The model under review builds one solid part; all positions refer to its coordinate system, in mm. Face numbers are marked on the shaded views. Coordinates: 2 decimals unless noted, no trailing zeros. Order: outer loops, then holes, each group sorted by start corner. A loop starts at its lowest first (then second) coordinate and runs counter-clockwise, first axis right, second up. Notation, with made-up numbers: M 80.25,65 L 126.25,65 A25 ccw 126.25,94 Z; hole C 52,82.25 d10. An arc over 180 degrees is marked long. Answer as CSV lines item,"result". Start each with the question number.
Q1. The part is to be moulded in two halves that separate along X. For the marked faces 1, 2 and 3, say which applies: +X half, -X half, draft (parallel to the pull), parting line (faces both ways), or undercut.
Q2. Wall thickness on L1, parallel to Y at x = -6.75, z = 19.5; L2, parallel to Y at x = 5.5, z = 7.25; L3, parallel to Y at x = -7.75, z = 26.25: over which ranges is each line inside the solid? List them lowest first. Write a range as [from, to].
Q3. Consider section C-C on z = 8.75. Write out the cut boundary in (x, y), and give its area (3 significant figures).
Q4. Consider section A-A on y = 0. Write out the cut boundary in (x, z), and give its area (3 significant figures).
Q5. For P1, Ø1.8, axis at x = 6.72, y = -6.72, coming from the -Z side, flat-tipped, find the tip position at first contact; note if it passes through.
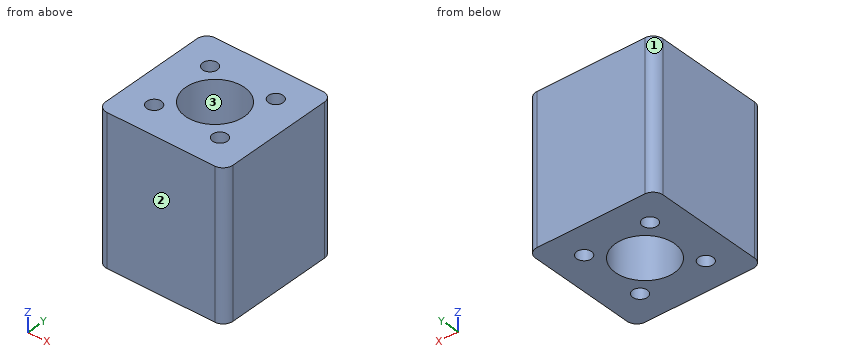
from build123d import *

# Parameters (mm, degrees)
SKETCH_1_R      = 1.5
SKETCH_1_R_2    = 6
EXTRUDE_1_DEPTH = 30


with BuildPart() as part:
    # 草图1 → 凸台-拉伸1 (new body)
    with BuildSketch(Plane.XY):
        with BuildLine():
            Line((0, 13), (11, 13))
            ThreePointArc((11, 13), (12.414213562, 12.414213562), (13, 11))
            Line((13, 11), (13, -11))
            ThreePointArc((13, -11), (12.414213562, -12.414213562), (11, -13))
            Line((11, -13), (-11, -13))
            ThreePointArc((-11, -13), (-12.414213562, -12.414213562), (-13, -11))
            Line((-13, -11), (-13, 11))
            ThreePointArc((-13, 11), (-12.414213562, 12.414213562), (-11, 13))
            Line((-11, 13), (0, 13))
        make_face()
        with Locations((-6.717514421, 6.717514421)):
            Circle(SKETCH_1_R, mode=Mode.SUBTRACT)
        with Locations((6.717514421, 6.717514421)):
            Circle(SKETCH_1_R, mode=Mode.SUBTRACT)
        with Locations((-6.717514421, -6.717514421)):
            Circle(SKETCH_1_R, mode=Mode.SUBTRACT)
        with Locations((6.717514421, -6.717514421)):
            Circle(SKETCH_1_R, mode=Mode.SUBTRACT)
        Circle(SKETCH_1_R_2, mode=Mode.SUBTRACT)
    extrude(amount=EXTRUDE_1_DEPTH)


solid = part.part
Evaluation:
1,face 1,"-X half"
1,face 2,"draft"
1,face 3,"undercut"
2,L1,"y = [-13, -8.22], [-5.22, 5.22], [8.22, 13]"
2,L2,"y = [-13, -7.59], [-5.84, -2.4], [2.4, 5.84], [7.59, 13]"
2,L3,"y = [-13, -7.81], [-5.63, 5.63], [7.81, 13]"
3,outline,"M -13,-11 A2 ccw -11,-13 L 11,-13 A2 ccw 13,-11 L 13,11 A2 ccw 11,13 L -11,13 A2 ccw -13,11 Z; hole C -6.72,-6.72 d3; hole C -6.72,6.72 d3; hole C 0,0 d12; hole C 6.72,-6.72 d3; hole C 6.72,6.72 d3"
3,area,"531 mm²"
4,outline,"M -13,0 L -6,0 L -6,30 L -13,30 Z; M 6,0 L 13,0 L 13,30 L 6,30 Z"
4,area,"420 mm²"
5,P1,"passes through"
